For this review, take the finished solid that the model builds, in its own axes (mm). Give positions to 0.01 mm unless a question says otherwise; leave off trailing zeros. Write each loop counter-clockwise with the first axis right and the second up, starting at its lowest first coordinate (ties: lowest second). Pieces come first, ordered by that corner, then holes.
1) We need section C-C on x = 5.5. Give the boundary of the cut face in (y, z), and give its area (3 significant figures).
2) Wall thickness on line 1 along Y through (x, z) = (0, 18); line 2 along X through (y, z) = (6.5, 16): over which ranges is each line inside the solid? List them lowest first.
3) For P1, Ø6, axis at y = 18, z = 24, coming from the +X side; P2, Ø1, axis at y = 21.5, z = 26, coming from the +X side; P3, Ø1.5, axis at x = 14.5, z = 15, coming from the +Y side, all flat-tipped, find the tip position at first contact; note any pin that passes through.
4) We need section D-D on z = 39. Give the boundary of the cut face in (x, y).
5) We need section A-A on z = 26. Give the boundary of the cut face in (x, y).
6) We need section B-B on y = 18. Give the boundary of the cut face in (x, z), and give its area (3 significant figures).
7) Draft analysis for pull direction Y (two halves, no side actions). For faces 1 (the face through (-4.986, -22.453, 19.177)), 2 (the face through (4, 23, 10)), 3 (the face through (12.92, -24.84, 20.29)), state which applies: pulls with the +Y half, pulls with the -Y half, needs draft (parallel to the pull), parting line crosses it, or undercut.
from build123d import *

# Parameters (mm, degrees)
CYLINDER015_R     = 28
CYLINDER015_DEPTH = 61
CYLINDER014_R     = 23
CYLINDER014_DEPTH = 38
CYLINDER013_R     = 28
CYLINDER013_DEPTH = 38
CYLINDER017_R     = 28
CYLINDER017_DEPTH = 61
CYLINDER016_R     = 23
CYLINDER016_DEPTH = 40
CYLINDER018_R     = 24
CYLINDER018_DEPTH = 40


with BuildPart() as cylinder015:
    # Cylinder015 → Cylinder015 (new body)
    with BuildSketch(Plane(origin=(-29, 0, 38), x_dir=(0, 0, -1), z_dir=(1, 0, 0))):
        Circle(CYLINDER015_R)
    extrude(amount=CYLINDER015_DEPTH)


with BuildPart() as cylinder014:
    # Cylinder014 → Cylinder014 (new body)
    with BuildSketch(Plane.XY):
        Circle(CYLINDER014_R)
    extrude(amount=CYLINDER014_DEPTH)


with BuildPart() as cut013:
    # Cylinder013 → Cylinder013 (new body)
    with BuildSketch(Plane.XY):
        Circle(CYLINDER013_R)
    extrude(amount=CYLINDER013_DEPTH)

    # Cut012: cut Cylinder014
    add(cylinder014.part, mode=Mode.SUBTRACT)

    # Cut013: cut Cylinder015
    add(cylinder015.part, mode=Mode.SUBTRACT)


with BuildPart() as cylinder017:
    # Cylinder017 → Cylinder017 (new body)
    with BuildSketch(Plane(origin=(-29, 0, 40), x_dir=(0, 0, -1), z_dir=(1, 0, 0))):
        Circle(CYLINDER017_R)
    extrude(amount=CYLINDER017_DEPTH)


with BuildPart() as cylinder016:
    # Cylinder016 → Cylinder016 (new body)
    with BuildSketch(Plane.XY):
        Circle(CYLINDER016_R)
    extrude(amount=CYLINDER016_DEPTH)


with BuildPart() as fusion002:
    # Cylinder018 → Cylinder018 (new body)
    with BuildSketch(Plane.XY):
        Circle(CYLINDER018_R)
    extrude(amount=CYLINDER018_DEPTH)

    # Cut014: cut Cylinder016
    add(cylinder016.part, mode=Mode.SUBTRACT)

    # Cut015: cut Cylinder017
    add(cylinder017.part, mode=Mode.SUBTRACT)

    # Fusion002: union Cut013
    add(cut013.part)


with BuildPart() as fusion002_1:
    # Fusion002 placement: moved
    add(fusion002.part.moved(Location((0, 0, 10))))


solid = fusion002_1.part
Results list:
1. outline: (-27.45, 10) - (-22.33, 10) - (-22.33, 33.11) arc R28 cw to (-23.36, 34.56) - (-23.36, 32.56) arc R28 cw to (-27.45, 42.5) - close; (22.33, 10) - (27.45, 10) - (27.45, 42.5) arc R28 cw to (23.36, 32.56) - (23.36, 34.56) arc R28 cw to (22.33, 33.11) - close
1. area: 267 mm2
2. line 1: y = -28 to -23, 23 to 28
2. line 2: x = -27.24 to -22.06, 22.06 to 27.24
3. P1: stops at x = 23.64
3. P2: stops at x = 18.52
3. P3: stops at y = 24.39
4. outline: (-9, -26.51) arc R28 ccw to (9, -26.51) - close; (-9, 26.51) - (9, 26.51) arc R28 ccw to start
5. outline: (-22, -17.32) arc R28 ccw to (22, -17.32) - (16.61, -17.32) arc R24 ccw to (19.18, -14.42) - (17.92, -14.42) arc R23 cw to (-17.92, -14.42) - (-19.18, -14.42) arc R24 ccw to (-16.61, -17.32) - close; (-22, 17.32) - (-16.61, 17.32) arc R24 ccw to (-19.18, 14.42) - (-17.92, 14.42) arc R23 cw to (17.92, 14.42) - (19.18, 14.42) arc R24 ccw to (16.61, 17.32) - (22, 17.32) arc R28 ccw to start
6. outline: (-21.45, 10) - (-14.32, 10) - (-14.32, 28.55) - (-15.87, 28.55) - (-15.87, 26.55) - (-21.45, 26.55) - close; (14.32, 10) - (21.45, 10) - (21.45, 26.55) - (15.87, 26.55) - (15.87, 28.55) - (14.32, 28.55) - close
6. area: 242 mm2
7. face 1: undercut
7. face 2: needs draft
7. face 3: parting line crosses it
